Input: part model. Units: mm. Frame: model coordinates. Face numbers are marked on the shaded views. A direction names the side the tool comes from. Give positions to 0.01 mm unless a question says otherwise; leave off trailing zeros. Loops run counter-clockwise (first coordinate to the right, second up) from the corner with the lowest first, then second, coordinate; pieces in that order, holes last. Notation, with made-up numbers: (-30.75, 51) -> (2.25, 51) arc R7 cw to (2.25, 56) -> close; hole circle Ø1 at (46, 24.5). An arc over 180 degrees is marked (long way). Answer as a JSON object with one key per item and string values.
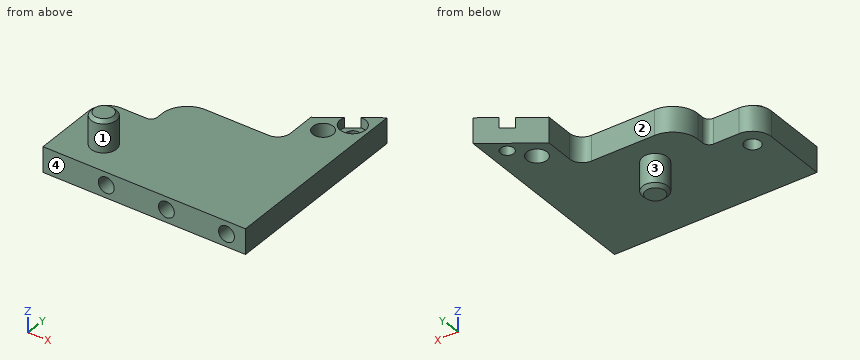
```python
from build123d import *

# Parameters (mm, degrees)
SKETCH1_W                       = 32
SKETCH1_H                       = 31.101660306
BOSS_EXTRUDE1_DEPTH             = 4
SKETCH2_W                       = 8
SKETCH2_H                       = 18.101660306
CUT_EXTRUDE1_DEPTH              = 5
SKETCH3_W                       = 16
SKETCH3_H                       = 12.101660306
CUT_EXTRUDE2_DEPTH              = 5
DRAFT1_ANGLE                    = -35.000000002
SKETCH4_W                       = 2
SKETCH4_H                       = 5
SKETCH5_W                       = 2
SKETCH5_H                       = 5
F_3_2_3_2_DIAMETER_HOLE1_D      = 3.2
F_3_2_3_2_DIAMETER_HOLE1_DEPTH  = 9
F_2_5_2_5_DIAMETER_HOLE1_D      = 2.5
F_2_5_2_5_DIAMETER_HOLE1_DEPTH  = 9
M4X0_7_TAPPED_HOLE1_D           = 2.1
M4X0_7_TAPPED_HOLE1_DEPTH       = 9
M4X0_7_TAPPED_HOLE1_CBORE_D     = 4
M4X0_7_TAPPED_HOLE1_CBORE_DEPTH = 1.6
F_2_5_2_5_DIAMETER_HOLE2_D      = 2.5
F_2_5_2_5_DIAMETER_HOLE2_DEPTH  = 7.5
F_2_5_2_5_DIAMETER_HOLE2_TIP    = 0.751075774
CHAMFER1_SIZE                   = 0.5
FILLET1_R                       = 1
FILLET2_R                       = 2
FILLET3_R                       = 3
FILLET4_R                       = 4


with BuildPart() as part:
    # Sketch1 → Boss-Extrude1 (new body)
    with BuildSketch(Plane(origin=(0, 0, 0), x_dir=(-1, 0, 0), z_dir=(0, 0, -1))):
        with Locations((-16, 15.550830153)):
            Rectangle(SKETCH1_W, SKETCH1_H)
    extrude(amount=-BOSS_EXTRUDE1_DEPTH)

    # Sketch2 → Cut-Extrude1 (cut, through all)
    with BuildSketch(Plane.XY.offset(4)):
        with Locations((4, 22.050830153)):
            Rectangle(SKETCH2_W, SKETCH2_H)
    extrude(amount=-CUT_EXTRUDE1_DEPTH, mode=Mode.SUBTRACT)

    # Sketch3 → Cut-Extrude2 (cut, through all)
    with BuildSketch(Plane.XY.offset(4)):
        with Locations((16, 25.050830153)):
            Rectangle(SKETCH3_W, SKETCH3_H)
    extrude(amount=-CUT_EXTRUDE2_DEPTH, mode=Mode.SUBTRACT)

    # Draft1
    draft1_faces = [part.faces().sort_by_distance(p)[0] for p in [
        (28, 31.101660306, 2),
    ]]
    draft(draft1_faces, Plane(origin=(32, 31.101660306, 4), x_dir=(0, 0, 1), z_dir=(1, 0, 0)), DRAFT1_ANGLE)

    # Sketch4 → Revolve1 (revolve)
    with BuildSketch(Plane.XZ.offset(-5)):
        with Locations((7, 6.5)):
            Rectangle(SKETCH4_W, SKETCH4_H)
    revolve(axis=Axis((6, 5, 9), (0, 0, -1)))

    # Sketch5 → Revolve2 (revolve)
    with BuildSketch(Plane(origin=(0, 14, 0), x_dir=(1, 0, 0), z_dir=(0, 1, 0))):
        with Locations((16.5, 2.5)):
            Rectangle(SKETCH5_W, SKETCH5_H)
    revolve(axis=Axis((15.5, 14, -5), (0, 0, 1)))

    # Ø3.2 (3.2) Diameter Hole1
    with Locations(Plane.XY.offset(4)):
        with Locations((27, 24)):
            Hole(F_3_2_3_2_DIAMETER_HOLE1_D / 2, depth=F_3_2_3_2_DIAMETER_HOLE1_DEPTH)

    # Ø2.5 (2.5) Diameter Hole1
    with Locations(Plane(origin=(0, 0, 0), x_dir=(-1, 0, 0), z_dir=(0, 0, -1))):
        with Locations((-3, 10)):
            Hole(F_2_5_2_5_DIAMETER_HOLE1_D / 2, depth=F_2_5_2_5_DIAMETER_HOLE1_DEPTH)

    # M4x0.7 Tapped Hole1
    with Locations(Plane.XY.offset(4)):
        with Locations((29.395995182, 27.202999702)):
            CounterBoreHole(M4X0_7_TAPPED_HOLE1_D / 2, M4X0_7_TAPPED_HOLE1_CBORE_D / 2, M4X0_7_TAPPED_HOLE1_CBORE_DEPTH, depth=M4X0_7_TAPPED_HOLE1_DEPTH)

    # Ø2.5 (2.5) Diameter Hole2
    with Locations(Plane(origin=(0, 0, 0), x_dir=(-1, 0, 0), z_dir=(0, -1, 0))):
        with Locations((-10, -2), (-19.5, -2), (-29, -2)):
            Hole(F_2_5_2_5_DIAMETER_HOLE2_D / 2, depth=F_2_5_2_5_DIAMETER_HOLE2_DEPTH)
            with Locations((0, 0, -(F_2_5_2_5_DIAMETER_HOLE2_DEPTH + F_2_5_2_5_DIAMETER_HOLE2_TIP / 2))):  # 118° drill point
                Cone(0, F_2_5_2_5_DIAMETER_HOLE2_D / 2, F_2_5_2_5_DIAMETER_HOLE2_TIP, mode=Mode.SUBTRACT)

    # Chamfer1
    chamfer1_edges = [part.edges().sort_by_distance(p)[0] for p in [
        (4, 5, 9),
        (13.5, 14, -5),
    ]]
    chamfer(chamfer1_edges, length=CHAMFER1_SIZE)

    # Fillet1
    fillet1_edges = [part.edges().sort_by_distance(p)[0] for p in [
        (8, 13, 2),
    ]]
    fillet(fillet1_edges, radius=FILLET1_R)

    # Fillet2
    fillet2_edges = [part.edges().sort_by_distance(p)[0] for p in [
        (24, 19, 2),
    ]]
    fillet(fillet2_edges, radius=FILLET2_R)

    # Fillet3
    fillet3_edges = [part.edges().sort_by_distance(p)[0] for p in [
        (0, 13, 2),
    ]]
    fillet(fillet3_edges, radius=FILLET3_R)

    # Fillet4
    fillet4_edges = [part.edges().sort_by_distance(p)[0] for p in [
        (8, 19, 2),
    ]]
    fillet(fillet4_edges, radius=FILLET4_R)


solid = part.part
```
Q1. Pin query (flat end, axial travel): pin 1 (3 mm diameter, centred on y = 7, z = -3, fed in from -X); pin 2 (2 mm diameter, centred on x = 19.5, z = 2, fed in from -Y); pin 3 (5 mm diameter, centred on x = 27, y = 24, fed in from -Z); pin 4 (1.1 mm diameter, centred on y = 14.5, z = 2, fed in from -X). Return the tip coordinate at first contact, or that it passes through.
Evaluation:
{"pin 1": "passes through", "pin 2": "stops at y = 7.65", "pin 3": "stops at z = 0", "pin 4": "stops at x = 8"}
Q2. Section B-B, the plane x = 6. Return the cut outline in (y, z), then the cut area to 4 significant figures.
Evaluation:
{"outline": "(0, 0) -> (13, 0) -> (13, 4) -> (7, 4) -> (7, 8.5) -> (6.5, 9) -> (3.5, 9) -> (3, 8.5) -> (3, 4) -> (0, 4) -> close", "area": "71.75 mm2"}
Q3. Section A-A, the plane y = 24. Return the cut outline in (x, z).
Evaluation:
{"outline": "(24, 0) -> (25.4, 0) -> (25.4, 4) -> (24, 4) -> close; (28.6, 0) -> (32, 0) -> (32, 4) -> (28.6, 4) -> close"}
Q4. Section D-D, the plane z = -2.25. Return the cut outline in (x, y), then the cut area to 3 significant figures.
Evaluation:
{"outline": "circle Ø4 at (15.5, 14)", "area": "12.6 mm2"}
Q5. Section C-C, the plane x = 27. Return the cut outline in (y, z), then the cut area to 3 significant figures.
Evaluation:
{"outline": "(0, 0) -> (22.4, 0) -> (22.4, 4) -> (0, 4) -> close; (25.6, 0) -> (27.6, 0) -> (27.6, 4) -> (25.6, 4) -> close", "area": "97.6 mm2"}
Q6. Ray query, line 1 along Z through (x, y) = (29, 2.5); line 2 along Y through (x, z) = (14, 2.5); line 3 along Z through (x, y) = (8, 4.5). Return the intervals inside material, ascending.
Evaluation:
{"line 1": "z = 0 to 0.75, 3.25 to 4", "line 2": "y = 0 to 19", "line 3": "z = 0 to 4"}
Q7. Access query for the marked faces 1, 2, 3 and 4. Directions: +Z, -Z, +X, -X, +Y, -Y. A direction counts if a zero-diameter tool reaches every point of the face in a straight line with its end or side. Return the directions, or none.
Evaluation:
{"face 1": "+Z", "face 2": "+Z, -Z, -X, +Y", "face 3": "-Z", "face 4": "+Z, -Z, +X, -X, -Y"}
